Can you work these out from the drawing? Everything is in mm from the part's minimum corner. Coordinates: 2 decimals unless noted, no trailing zeros. Write each loop counter-clockwise with the first axis right and the second up, starting at its lowest first coordinate (ties: lowest second). Pieces come first, ordered by that corner, then holes.
(1) Imagine slicing it at C-C, the plane z = 168.5. List the corners of the cut face in (x, y) for me (1 decimal).
(2) Imagine slicing it at D-D, the plane z = 105. List the corners of the cut face in (x, y) for me.
(3) Imagine slicing it at A-A, the plane x = 14. List the corners of the cut face in (y, z) for me.
(4) Imagine slicing it at B-B, the plane y = 4.2. State how many separate pieces and enclosed holes the cut face has, plus the area to 3 significant figures.
(5) Please list where these lines run through material, in increasing order: probe 1 along Z at (x, y) = (20.5, 3.9); probe 2 along Z at (x, y) = (19, 2.85); probe 3 along X at (y, z) = (1.15, 163).
(6) For pin 1 Ø3.5 at (x, z) = (60.55, 168.5) entering from -Y; pin 2 Ø1.5 at (x, y) = (28.5, 3) entering from +Z; pin 3 Ø1 at (y, z) = (1, 111.5) entering from +X; pin 4 Ø1.5 at (x, y) = (49.5, 1) entering from -Z, each with a flat end and sliding along its axis, tell me the tip position at first contact or that it passes through.
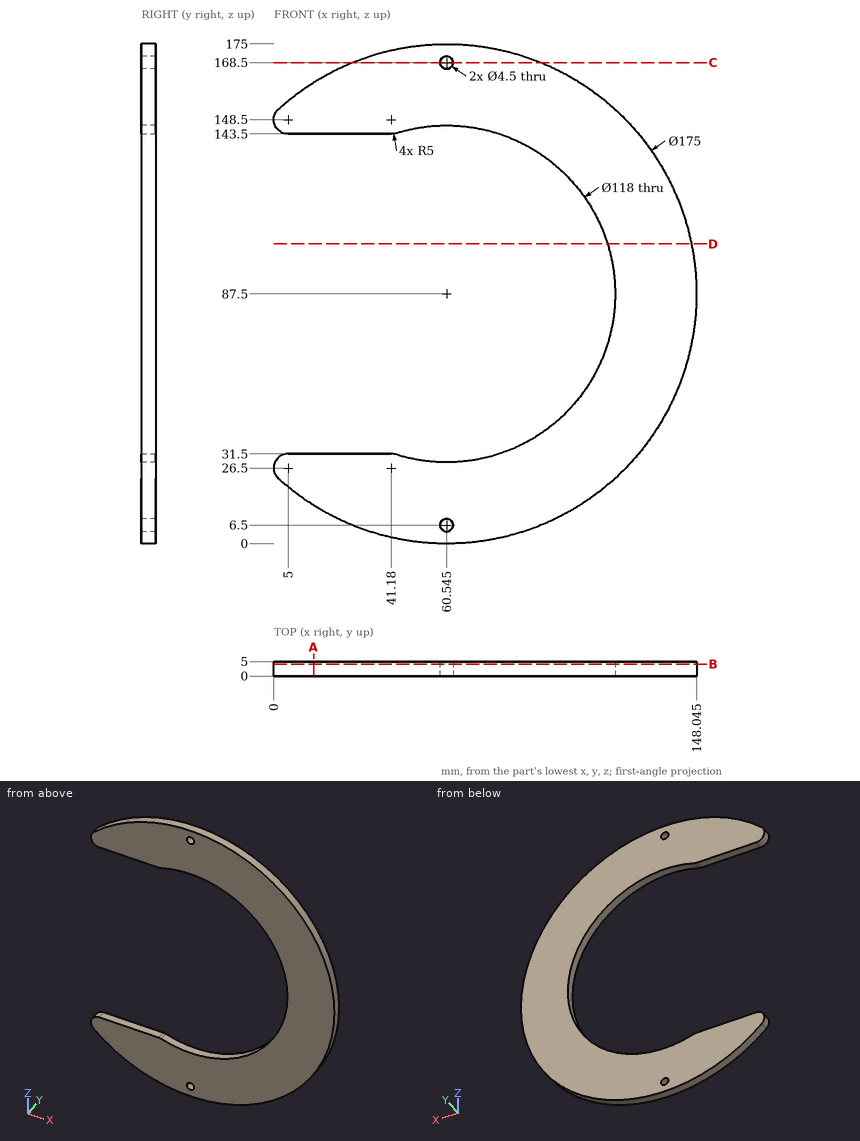
Recorded:
1. outline: (27.5, 0) - (58.3, 0) - (58.3, 5) - (27.5, 5) - close; (62.8, 0) - (93.6, 0) - (93.6, 5) - (62.8, 5) - close
2. outline: (116.89, 0) - (146.28, 0) - (146.28, 5) - (116.89, 5) - close
3. outline: (0, 13.41) - (5, 13.41) - (5, 31.5) - (0, 31.5) - close; (0, 143.5) - (5, 143.5) - (5, 161.59) - (0, 161.59) - close
4. separate pieces: 1
4. enclosed holes: 2
4. area: 9,330 mm2
5. probe 1: z = 9.7 to 31.5, 143.5 to 165.3
5. probe 2: z = 10.49 to 31.5, 143.5 to 164.51
5. probe 3: x = 16.32 to 104.77
6. pin 1: passes through
6. pin 2: stops at z = 169.21
6. pin 3: stops at x = 144.83
6. pin 4: stops at z = 0.61
